Build history of the part. All positions in model axes, mm. Coordinates: 2 decimals unless noted, no trailing zeros. Loops run counter-clockwise (first coordinate to the right, second up) from the corner with the lowest first, then second, coordinate; pieces in that order, holes last. Notation, with made-up numbers: (58.5, 9.25) -> (94.5, 9.25) arc R24 ccw to (94.5, 24.25) -> close; hole circle Ø5 at (81, 49.5). An arc over 180 degrees is marked (long way). One line per item, written item: value. Start each with the question number.
```python
from build123d import *

# Parameters (mm, degrees)
SKETCH2_W           = 300
SKETCH2_H           = 50
BOSS_EXTRUDE1_DEPTH = 31.75
SKETCH3_R           = 4.8
SKETCH3_R_2         = 2.25
CUT_EXTRUDE1_DEPTH  = 31.75
SKETCH3_3_R         = 2.25
CUT_EXTRUDE2_DEPTH  = 31.75


with BuildPart() as part:
    # Sketch2 → Boss-Extrude1 (new body)
    with BuildSketch(Plane(origin=(0, 0, 0), x_dir=(1, 0, 0), z_dir=(0, 1, 0))):
        with Locations((150, 25)):
            Rectangle(SKETCH2_W, SKETCH2_H)
    extrude(amount=BOSS_EXTRUDE1_DEPTH)

    # Sketch3 → Cut-Extrude1 (cut)
    with BuildSketch(Plane(origin=(0, 31.75, 0), x_dir=(1, 0, 0), z_dir=(0, 1, 0))):
        with Locations(Location((30, 25, 0), (0, 0, 270))):
            Circle(SKETCH3_R)
        with Locations(Location((270, 25, 0), (0, 0, 270))):
            Circle(SKETCH3_R)
        with Locations(Location((22.5, 19, 0), (0, 0, 270))):
            Circle(SKETCH3_R_2)
        with Locations(Location((277.5, 19, 0), (0, 0, 270))):
            Circle(SKETCH3_R_2)
    extrude(amount=-CUT_EXTRUDE1_DEPTH, mode=Mode.SUBTRACT)

    # Sketch3_3 → Cut-Extrude2 (cut)
    with BuildSketch(Plane(origin=(0, 31.75, 0), x_dir=(1, 0, 0), z_dir=(0, 1, 0))):
        with Locations(Location((37.5, 31, 0), (0, 0, 270))):
            Circle(SKETCH3_3_R)
        with Locations(Location((37.5, 19, 0), (0, 0, 270))):
            Circle(SKETCH3_3_R)
        with Locations(Location((22.5, 31, 0), (0, 0, 270))):
            Circle(SKETCH3_3_R)
        with Locations(Location((277.5, 31, 0), (0, 0, 270))):
            Circle(SKETCH3_3_R)
        with Locations(Location((262.5, 19, 0), (0, 0, 270))):
            Circle(SKETCH3_3_R)
        with Locations(Location((262.5, 31, 0), (0, 0, 270))):
            Circle(SKETCH3_3_R)
    extrude(amount=-CUT_EXTRUDE2_DEPTH, mode=Mode.SUBTRACT)


solid = part.part
```
Item 1: Two-plate mould, pull along Z, no slides. Class faces 1 (the face through (274.76, 16.1, -25.62)), 2 (the face through (0, 16, -25)), 3 (the face through (148, 16, -50)): +Z half, -Z half, draft (parallel to the pull), parting line (faces both ways), or undercut.
Item 2: Drop flat-ended pins along their axis: pin 1 Ø3.5 at (x, z) = (37.5, -31) entering from -Y; pin 2 Ø6 at (x, z) = (262.5, -31) entering from -Y. Give the stop position or say it passes through.
Item 3: Band-saw the part on A-A, the plane x = 270. List the corners of the cut face in (y, z), and give its area (3 significant figures).
Item 4: Band-saw the part on B-B, the plane y = 4.5. Count the separate pieces of the cut face and the enclosed holes in it, and give its area (3 significant figures).
Item 5: Probe probe 1 along Z at (x, y) = (262, 13); probe 2 along X at (y, z) = (10, -25); probe 3 along X at (y, z) = (7, -31). List the from-to ranges inside material, lowest first.
Worked out:
1. face 1: undercut
1. face 2: draft
1. face 3: -Z half
2. pin 1: passes through
2. pin 2: stops at y = 0
3. outline: (0, -50) -> (31.75, -50) -> (31.75, -29.8) -> (0, -29.8) -> close; (0, -20.2) -> (31.75, -20.2) -> (31.75, 0) -> (0, 0) -> close
3. area: 1,280 mm²
4. separate pieces: 1
4. enclosed holes: 10
4. area: 14,700 mm²
5. probe 1: z = -50 to -33.19, -28.81 to -21.19, -16.81 to 0
5. probe 2: x = 0 to 25.2, 34.8 to 265.2, 274.8 to 300
5. probe 3: x = 0 to 20.25, 24.75 to 35.25, 39.75 to 260.25, 264.75 to 275.25, 279.75 to 300
